Job drawing, mm, ordinate dimensions from the low corner. One solid piece. A direction names the side the tool comes from. Give positions to 0.01 mm unless a question says otherwise; leave off trailing zeros. Write each loop counter-clockwise with the first axis right and the second up, starting at its lowest first coordinate (ties: lowest second). Pieces come first, ordered by that corner, then holes. Notation, with made-up numbers: (55, 64.25) - (114, 64.25) arc R22 ccw to (114, 98.25) - close; hole circle Ø2 at (56, -19). An arc over 180 degrees is marked (long way). Answer as a JSON object with one key per item and string values.
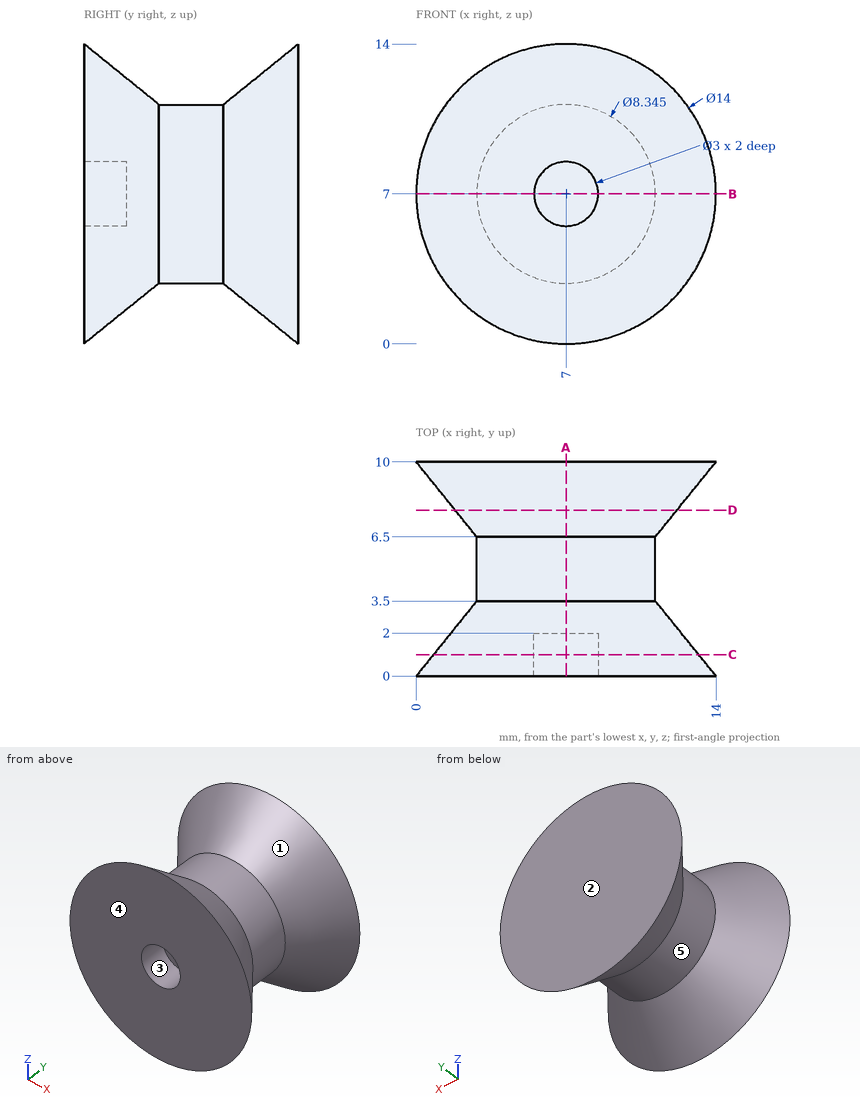
Item 1: Flat gauge pins, fed straight in: P1, Ø1.8, axis at x = 7, z = 7, coming from the -Y side; P2, Ø1, axis at y = 3.5, z = 10.5, coming from the -X side. Where does each tip first touch, or does it go through?
Entries:
{"P1": "y = 2", "P2": "x = 3.84"}
Item 2: Which spindle directions (+Z, -Z, +X, -X, +Y, -Y) get a long thin tool onto all of the face, cutting with end or side? Do the marked faces 1 and 2. Say none if no direction does.
Entries:
{"face 1": "none", "face 2": "+Z, -Z, +X, -X, +Y"}
Item 3: Cut at B-B (z = 7). Give the cut face in (x, y).
Entries:
{"outline": "(0, 0) - (5.5, 0) - (5.5, 2) - (8.5, 2) - (8.5, 0) - (14, 0) - (11.17, 3.5) - (11.17, 6.5) - (14, 10) - (0, 10) - (2.83, 6.5) - (2.83, 3.5) - close"}
Item 4: Probe line 1 (Z direction, x = 7, y = 1.05); line 2 (X direction, y = 0.75, z = 7); line 3 (Z direction, x = 7, y = 0.7) (1 decimal). List the from-to ranges inside material, lowest first. Write a range as from..to.
Entries:
{"line 1": "0.85..5.5, 8.5..13.15", "line 2": "0.61..5.5, 8.5..13.39", "line 3": "0.6..5.5, 8.5..13.4"}
Item 5: Cut at C-C (y = 1). Give the cut face in (x, z), and give its area (3 significant figures).
Entries:
{"outline": "circle Ø12.38 at (7, 7); hole circle Ø3 at (7, 7)", "area": "113 mm2"}
Item 6: Mould opens along X. For the marked faces 3, 4 and 5 say: +X half, -X half, draft (parallel to the pull), parting line (faces both ways), or undercut.
Entries:
{"face 3": "undercut", "face 4": "draft", "face 5": "parting line"}
Item 7: Cut at A-A (x = 7). Give the cut face in (y, z).
Entries:
{"outline": "(0, 0) - (3.5, 2.83) - (6.5, 2.83) - (10, 0) - (10, 14) - (6.5, 11.17) - (3.5, 11.17) - (0, 14) - (0, 8.5) - (2, 8.5) - (2, 5.5) - (0, 5.5) - close"}
Item 8: Cut at D-D (y = 7.75). Give the cut face in (x, z).
Entries:
{"outline": "circle Ø10.36 at (7, 7)"}
